from build123d import *

# Parameters (mm, degrees)
F0_R     = 25.4
F0_R_2   = 5.207
F1_DEPTH = 6.35


with BuildPart() as f1:
    # F0 (on Front) → F1 (new body)
    with BuildSketch(Plane.XZ):
        Circle(F0_R)
        with BuildLine():
            ThreePointArc((19.2474145991, 11.1125), (21.4677014893, 5.7522532774), (22.225, 0))
            ThreePointArc((22.225, 0), (21.4677014893, -5.7522532774), (19.2474145991, -11.1125))
            ThreePointArc((19.2474145991, -11.1125), (15.7154482119, -15.7154482119), (11.1125, -19.2474145991))
            ThreePointArc((11.1125, -19.2474145991), (5.7522532774, -21.4677014893), (0, -22.225))
            ThreePointArc((0, -22.225), (-5.7522532774, -21.4677014893), (-11.1125, -19.2474145991))
            ThreePointArc((-11.1125, -19.2474145991), (-15.7154482119, -15.7154482119), (-19.2474145991, -11.1125))
            ThreePointArc((-19.2474145991, -11.1125), (-21.4677014893, -5.7522532774), (-22.225, 0))
            ThreePointArc((-22.225, 0), (-21.4677014893, 5.7522532774), (-19.2474145991, 11.1125))
            ThreePointArc((-19.2474145991, 11.1125), (-15.7154482119, 15.7154482119), (-11.1125, 19.2474145991))
            ThreePointArc((-11.1125, 19.2474145991), (-5.7522532774, 21.4677014893), (0, 22.225))
            ThreePointArc((0, 22.225), (5.7522532774, 21.4677014893), (11.1125, 19.2474145991))
            ThreePointArc((11.1125, 19.2474145991), (15.7154482119, 15.7154482119), (19.2474145991, 11.1125))
        make_face(mode=Mode.SUBTRACT)
        with BuildLine():
            ThreePointArc((6.5991135768, -3.81), (7.3603547963, -1.9722011237), (7.62, 0))
            ThreePointArc((7.62, 0), (7.3603547963, 1.9722011237), (6.5991135768, 3.81))
            ThreePointArc((6.5991135768, 3.81), (5.3881536726, 5.3881536726), (3.81, 6.5991135768))
            ThreePointArc((3.81, 6.5991135768), (1.9722011237, 7.3603547963), (0, 7.62))
            ThreePointArc((0, 7.62), (-1.9722011237, 7.3603547963), (-3.81, 6.5991135768))
            ThreePointArc((-3.81, 6.5991135768), (-5.3881536726, 5.3881536726), (-6.5991135768, 3.81))
            ThreePointArc((-6.5991135768, 3.81), (-7.3603547963, 1.9722011237), (-7.62, 0))
            ThreePointArc((-7.62, 0), (-7.3603547963, -1.9722011237), (-6.5991135768, -3.81))
            ThreePointArc((-6.5991135768, -3.81), (-5.3881536726, -5.3881536726), (-3.81, -6.5991135768))
            ThreePointArc((-3.81, -6.5991135768), (-1.9722011237, -7.3603547963), (0, -7.62))
            ThreePointArc((0, -7.62), (1.9722011237, -7.3603547963), (3.81, -6.5991135768))
            ThreePointArc((3.81, -6.5991135768), (5.3881536726, -5.3881536726), (6.5991135768, -3.81))
        make_face()
        Circle(F0_R_2, mode=Mode.SUBTRACT)
        with BuildLine():
            Line((6.5991135768, 3.81), (19.2474145991, 11.1125))
            ThreePointArc((19.2474145991, 11.1125), (15.7154482119, 15.7154482119), (11.1125, 19.2474145991))
            Line((11.1125, 19.2474145991), (3.81, 6.5991135768))
            ThreePointArc((3.81, 6.5991135768), (5.3881536726, 5.3881536726), (6.5991135768, 3.81))
        make_face()
        with BuildLine():
            Line((0, 7.62), (0, 22.225))
            ThreePointArc((0, 22.225), (-5.7522532774, 21.4677014893), (-11.1125, 19.2474145991))
            Line((-11.1125, 19.2474145991), (-3.81, 6.5991135768))
            ThreePointArc((-3.81, 6.5991135768), (-1.9722011237, 7.3603547963), (0, 7.62))
        make_face()
        with BuildLine():
            Line((-6.5991135768, 3.81), (-19.2474145991, 11.1125))
            ThreePointArc((-19.2474145991, 11.1125), (-21.4677014893, 5.7522532774), (-22.225, 0))
            Line((-22.225, 0), (-7.62, 0))
            ThreePointArc((-7.62, 0), (-7.3603547963, 1.9722011237), (-6.5991135768, 3.81))
        make_face()
        with BuildLine():
            ThreePointArc((-19.2474145991, -11.1125), (-15.7154482119, -15.7154482119), (-11.1125, -19.2474145991))
            Line((-11.1125, -19.2474145991), (-3.81, -6.5991135768))
            ThreePointArc((-3.81, -6.5991135768), (-5.3881536726, -5.3881536726), (-6.5991135768, -3.81))
            Line((-6.5991135768, -3.81), (-19.2474145991, -11.1125))
        make_face()
        with BuildLine():
            ThreePointArc((0, -22.225), (5.7522532774, -21.4677014893), (11.1125, -19.2474145991))
            Line((11.1125, -19.2474145991), (3.81, -6.5991135768))
            ThreePointArc((3.81, -6.5991135768), (1.9722011237, -7.3603547963), (0, -7.62))
            Line((0, -7.62), (0, -22.225))
        make_face()
        with BuildLine():
            ThreePointArc((19.2474145991, -11.1125), (21.4677014893, -5.7522532774), (22.225, 0))
            Line((22.225, 0), (7.62, 0))
            ThreePointArc((7.62, 0), (7.3603547963, -1.9722011237), (6.5991135768, -3.81))
            Line((6.5991135768, -3.81), (19.2474145991, -11.1125))
        make_face()
    extrude(amount=F1_DEPTH)


solid = f1.part
Design review of the part built by this model. Coordinates are the model's own, in mm. Give positions to 0.01 mm unless a question says otherwise; leave off trailing zeros. Order: outer loops, then holes, each group sorted by start corner. A loop starts at its lowest first (then second) coordinate and runs counter-clockwise, first axis right, second up. Notation, with made-up numbers: (59.5, 18.25) - (74.5, 18.25) arc R19 cw to (74.5, 22.25) - close; hole circle Ø7 at (-33, 1). An arc over 180 degrees is marked (long way). Write item = value, one per line. Start each with the question number.
Q1. Mouldability with a two-part tool opening along X and no side actions: class faces 1 (the face through (-6, 0, 0)), 2 (the face through (0, -3, 15)), 3 (the face through (-5.506, -3.131, -24.796)) as released by +X, released by -X, zero draft, split by the parting line, or undercut.
Q2. Clearance check with flat-ended pins moving along their axes: pin 1 Ø3 at (x, y) = (-17, -1.5) entering from -Z; pin 2 Ø12 at (x, z) = (11.5, -14.5) entering from +Y; pin 3 Ø2 at (x, y) = (6.5, -1.5) entering from -Z; pin 4 Ø3 at (y, z) = (-5, 14.5) entering from +X. State where each tip first meets the part, or that it passes through.
Q3. We need section A-A on y = -4.25. State how many separate pieces and enclosed holes the cut face has, plus the area to 3 significant figures.
Q4. We need section D-D on z = 15. State the section outline as (x, y) points, plus the area to 3 significant figures.
Q5. We need section C-C on z = 4.5. State the section outline as (x, y) points, plus the area to 3 significant figures.
Q6. We need section B-B on x = -17. State the section outline as (y, z) points.
Q7. To check wall thickness, follow L1, parallel to Z at x = 12.5, y = -2; L2, parallel to Z at x = -15.5, y = -2; L3, parallel to Z at x = -4, y = -3.75. State the ranges of each line that lie inside material, in increasing order. Write a range as from..to.
Working result:
q1.face_1 = zero draft
q1.face_2 = undercut
q1.face_3 = split by the parting line
q2.pin_1 = -20.12
q2.pin_2 = 0
q2.pin_3 = -24.8
q2.pin_4 = 21.82
q3.separate_pieces = 1
q3.enclosed_holes = 7
q3.area = 1,260 mm²
q4.outline = (-20.5, -6.35) - (-16.4, -6.35) - (-16.4, 0) - (-20.5, 0) - close; (-8.66, -6.35) - (0, -6.35) - (0, 0) - (-8.66, 0) - close; (8.66, -6.35) - (20.5, -6.35) - (20.5, 0) - (8.66, 0) - close
q4.area = 156 mm²
q5.outline = (-25, -6.35) - (-7.79, -6.35) - (-7.79, 0) - (-25, 0) - close; (-6.15, -6.35) - (-2.62, -6.35) - (-2.62, 0) - (-6.15, 0) - close; (2.62, -6.35) - (7.79, -6.35) - (7.79, 0) - (2.62, 0) - close; (21.76, -6.35) - (25, -6.35) - (25, 0) - (21.76, 0) - close
q5.area = 185 mm²
q6.outline = (-6.35, -18.87) - (0, -18.87) - (0, -9.81) - (-6.35, -9.81) - close; (-6.35, 0) - (0, 0) - (0, 9.81) - (-6.35, 9.81) - close; (-6.35, 14.32) - (0, 14.32) - (0, 18.87) - (-6.35, 18.87) - close
q7.L1 = -22.11..-18.38, -7.22..0, 7.22..22.11
q7.L2 = -20.12..-8.95, 0..8.95, 15.93..20.12
q7.L3 = -25.08..-21.86, -6.93..-3.33, 3.33..6.49, 6.93..25.08
